from build123d import *

# Parameters (mm, degrees)
F0_R     = 35.1
F0_R_2   = 34.5
F1_DEPTH = 5
F0_R_3   = 33.6999967694
F0_R_4   = 33.0999977887
F3_R     = 34.5
F3_R_2   = 33.6999967694
F4_DEPTH = 0.075


with BuildPart() as f1:
    # F0 (on Front) → F1 (new body)
    with BuildSketch(Plane.XZ):
        Circle(F0_R)
        Circle(F0_R_2, mode=Mode.SUBTRACT)
    extrude(amount=F1_DEPTH)



with BuildPart() as f1b:
    # F0 (on Front) → F1, piece 2 (new body)
    with BuildSketch(Plane.XZ):
        Circle(F0_R_3)
        Circle(F0_R_4, mode=Mode.SUBTRACT)
    extrude(amount=F1_DEPTH)


with BuildPart() as f1_1:
    add(f1.part)

    add(f1b.part)  # F4 merges F1b
    # F3 (on offset) → F4 (join, symmetric)
    with BuildSketch(Plane.XZ.offset(2.5)):
        Circle(F3_R)
        Circle(F3_R_2, mode=Mode.SUBTRACT)
    extrude(amount=F4_DEPTH, both=True)


solid = f1_1.part
Model file for the job. Use its own axes, mm. A direction names the side the tool comes from. Give positions to 0.01 mm unless a question says otherwise; leave off trailing zeros. Loops run counter-clockwise (first coordinate to the right, second up) from the corner with the lowest first, then second, coordinate; pieces in that order, holes last.
Item 1: Drill centre lines: line 1 along Z through (x, y) = (0, -3.2); line 2 along Z through (x, y) = (5, -0.8); line 3 along X through (y, z) = (-1.25, -2). Where is each one in solid material? Low to high.
Check values:
line 1: z = -35.1 to -34.5, -33.7 to -33.1, 33.1 to 33.7, 34.5 to 35.1
line 2: z = -34.74 to -34.14, -33.33 to -32.72, 32.72 to 33.33, 34.14 to 34.74
line 3: x = -35.04 to -34.44, -33.64 to -33.04, 33.04 to 33.64, 34.44 to 35.04
Item 2: Slice it at C-C (x = -16). Write the cut outline in (y, z) (1 decimal).
Check values:
outline: (-5, -31.2) - (0, -31.2) - (0, -30.6) - (-2.4, -30.6) - (-2.4, -29.7) - (0, -29.7) - (0, -29) - (-5, -29) - (-5, -29.7) - (-2.6, -29.7) - (-2.6, -30.6) - (-5, -30.6) - close; (-5, 29) - (0, 29) - (0, 29.7) - (-2.4, 29.7) - (-2.4, 30.6) - (0, 30.6) - (0, 31.2) - (-5, 31.2) - (-5, 30.6) - (-2.6, 30.6) - (-2.6, 29.7) - (-5, 29.7) - close
Item 3: Mould opens along X. For faces 1 (the face through (23, 0, -26)), 2 (the face through (8, -2.425, -33)), 3 (the face through (-27.85, -2.46, -21.36)) say: +X half, -X half, draft (parallel to the pull), parting line (faces both ways), or undercut.
Check values:
face 1: draft
face 2: undercut
face 3: parting line
Item 4: Which spindle directions (+Z, -Z, +X, -X, +Y, -Y) get a long thin tool onto all of the face, cutting with end or side? Do faces 4 (the face through (8, -2.575, -33)), 5 (the face through (-7.3, -1.2, -32.9)), 6 (the face through (23, -5, -26)). Say none if no direction does.
Check values:
face 4: -Y
face 5: +Y
face 6: +Z, -Z, +X, -X, -Y
Item 5: Drop a flat-ended pin along its axis: P1, Ø1.5, axis at x = 23.5, z = -21.5, coming from the -Y side (1 decimal). Give the stop position or say it passes through.
Check values:
P1: passes through
Item 6: Slice it at B-B (y = -1.35). Write the cut outline in (x, z), plus the area to 3 significant figures.
Check values:
outline: circle Ø70.2 at (0, 0); circle Ø67.4 at (0, 0); hole circle Ø69 at (0, 0); hole circle Ø66.2 at (0, 0)
area: 257 mm2
Item 7: Slice it at A-A (z = 0). Write the cut outline in (x, y) (3 decimals), plus the area to 3 significant figures.
Check values:
outline: (-35.1, -5) - (-34.5, -5) - (-34.5, -2.575) - (-33.7, -2.575) - (-33.7, -5) - (-33.1, -5) - (-33.1, 0) - (-33.7, 0) - (-33.7, -2.425) - (-34.5, -2.425) - (-34.5, 0) - (-35.1, 0) - close; (33.1, -5) - (33.7, -5) - (33.7, -2.575) - (34.5, -2.575) - (34.5, -5) - (35.1, -5) - (35.1, 0) - (34.5, 0) - (34.5, -2.425) - (33.7, -2.425) - (33.7, 0) - (33.1, 0) - close
area: 12.2 mm2
